Part model, mm, in its own coordinate system. A direction names the side the tool comes from. Give positions to 0.01 mm unless a question says otherwise; leave off trailing zeros. Write each loop counter-clockwise with the first axis right and the second up, starting at its lowest first coordinate (ties: lowest second). Pieces come first, ordered by that corner, then holes. Notation, with made-up numbers: (-17.75, 47) - (-0.75, 47) arc R16 cw to (-0.75, 60) - close; hole circle Ø6 at (-16.75, 21). An arc over 180 degrees is marked (long way). Answer as a JSON object with one key per item and string values. Group by question number.
```python
from build123d import *

# Parameters (mm, degrees)
F1_DEPTH = 63.5
F2_DEPTH = 25.4
F3_DEPTH = 7.9375
F0_W     = 25.4
F0_H     = 19.05
F4_DEPTH = 25.4
F6_R     = 6.35
F7_R     = 6.35


with BuildPart() as f1:
    # F0 (on Front) → F1 (new body, symmetric)
    with BuildSketch(Plane.XZ):
        Polygon((-41.275, 9.525), (-41.275, -9.525), (41.275, -9.525), (41.275, 9.525), (22.225, 9.525), align=None)
    extrude(amount=F1_DEPTH, both=True)

    # F0 (on Front) → F2 (join, symmetric)
    with BuildSketch(Plane.XZ):
        with BuildLine():
            Line((22.225, 9.525), (41.275, 9.525))
            Line((41.275, 9.525), (41.275, 27.0002))
            ThreePointArc((41.275, 27.0002), (45.9246798487, 38.2255201513), (57.15, 42.8752))
            Line((57.15, 42.8752), (60.325, 42.8752))
            Line((60.325, 42.8752), (60.325, 61.9252))
            Line((60.325, 61.9252), (57.15, 61.9252))
            add(Edge.make_bspline(
                [(53.9637073278, 61.7795496777), (55.021415818, 61.8378973507), (56.0835450938, 61.8864198253), (57.15, 61.9252)],
                knots=[108.6046989527, 108.6046989527, 108.6046989527, 108.6046989527, 111.5045361635, 111.5045361635, 111.5045361635, 111.5045361635], degree=3))
            ThreePointArc((53.9637073278, 61.7795496777), (31.3523557609, 50.5424423892), (22.225, 27.0002))
            Line((22.225, 27.0002), (22.225, 9.525))
        make_face()
    extrude(amount=F2_DEPTH, both=True)

    # F0 (on Front) → F3 (join, symmetric)
    with BuildSketch(Plane.XZ):
        with BuildLine():
            add(Edge.make_bspline(
                [(-41.275, 9.525), (-19.0620616146, 43.6277397004), (14.35041051, 59.5943127151), (53.9637073278, 61.7795496777)],
                knots=[0, 0, 0, 0, 108.6046989527, 108.6046989527, 108.6046989527, 108.6046989527], degree=3))
            Line((-41.275, 9.525), (22.225, 9.525))
            Line((22.225, 9.525), (22.225, 27.0002))
            ThreePointArc((22.225, 27.0002), (31.3523557609, 50.5424423892), (53.9637073278, 61.7795496777))
        make_face()
    extrude(amount=F3_DEPTH, both=True)

    # F0 (on Front) → F4 (join, symmetric)
    with BuildSketch(Plane.XZ):
        with Locations((73.025, 52.4002)):
            Rectangle(F0_W, F0_H)
    extrude(amount=F4_DEPTH, both=True)

    # F0 (on Front) → F5 (revolve)
    with BuildSketch(Plane.XZ):
        Polygon((85.725, 66.675), (85.725, 61.9252), (85.725, 42.8752), (85.725, 38.1), (111.125, 38.1), (111.125, 66.675), align=None)
    revolve(axis=Axis((85.725, 0, 52.3875), (0, 0, 1)))

    # F6
    f6_edges = [f1.edges().sort_by_distance(p)[0] for p in [
        (-41.275, -63.5, 0),
        (41.275, -63.5, 0),
        (41.275, 63.5, 0),
    ]]
    fillet(f6_edges, radius=F6_R)

    # F7
    f7_edges = [f1.edges().sort_by_distance(p)[0] for p in [
        (-41.275, 63.5, 0),
    ]]
    fillet(f7_edges, radius=F7_R)


solid = f1.part
```
1) Two-plate mould, pull along X, no slides. Class faces 1 (the flat face through (-41.275, -1, 0)), 2 (the cylindrical face through (45.8, -0.4, 38.1)), 3 (the flat face through (46, -25.4, 42)), 4 (the flat face through (41.275, -1, 4)): +X half, -X half, draft (parallel to the pull), parting line (faces both ways), or undercut.
2) Drop flat-ended pins along their axis: P1, Ø15.5, axis at x = 14.5, z = 31, coming from the +Y side; P2, Ø8.5, axis at y = -20.5, z = 20, coming from the -X side (3 decimals); P3, Ø6, axis at x = 0, y = 26.5, coming from the +Z side (3 decimals). Give the stop position or say it passes through.
3) Which spindle directions (+Z, -Z, +X, -X, +Y, -Y) get a long thin tool onto all of the face, cutting with end or side? Do faces 5 (the flat face through (86, 0, 38.1)), 6 (the flat face through (22.225, 17, 18)), 7 (the flat face through (22.225, -17, 18)). Say none if no direction does.
4) Saw through at B-B (y = 44.5). List the corners of the cut face in (x, z) (3 decimals), and give its area (3 significant figures).
5) Drill centre lines: line 1 along Z through (x, y) = (15, 25.5) (3 decimals); line 2 along Y through (x, z) = (-2.5, 15); line 3 along Y through (x, z) = (77, 49). Where is each one in solid material? Low to high. Write a range as from..to.
6) Saw through at A-A (x = 78.5). List the corners of the cut face in (y, z) (3 decimals).
Checks:
{
 "1": {"face 1": "-X half", "face 2": "undercut", "face 3": "draft", "face 4": "+X half"},
 "2": {"P1": "y = 7.94", "P2": "x = 22.225", "P3": "z = 9.525"},
 "3": {"face 5": "-Z, +X, +Y, -Y", "face 6": "+Z, -X, +Y", "face 7": "+Z, -X, -Y"},
 "4": {"outline": "(-41.275, -9.525) - (41.275, -9.525) - (41.275, 9.525) - (-41.275, 9.525) - close", "area": "1,570 mm2"},
 "5": {"line 1": "-9.525..9.525", "line 2": "-7.94..7.94", "line 3": "-25.4..25.4"},
 "6": {"outline": "(-25.4, 42.875) - (-24.351, 42.875) - (-24.351, 38.1) - (24.351, 38.1) - (24.351, 42.875) - (25.4, 42.875) - (25.4, 61.925) - (24.351, 61.925) - (24.351, 66.675) - (-24.351, 66.675) - (-24.351, 61.925) - (-25.4, 61.925) - close"}
}
